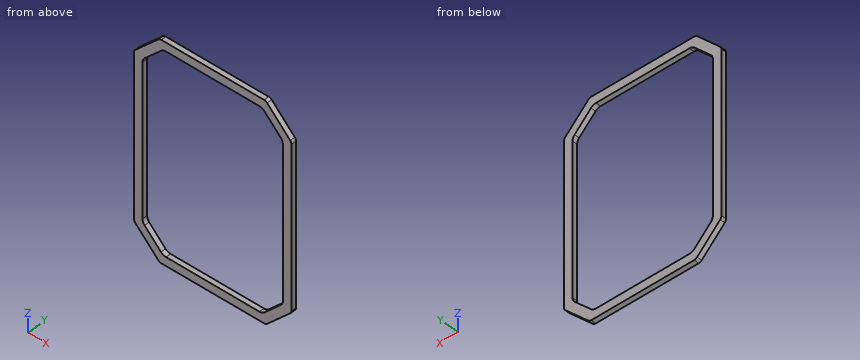
```python
from build123d import *

# Parameters (mm, degrees)
BOSS_EXTRUDE1_DEPTH = 1.75


with BuildPart() as part:
    # Sketch1 → Boss-Extrude1 (new body)
    with BuildSketch(Plane(origin=(-905.783657891, 0, -1752.480725949), x_dir=(1, 0, 0), z_dir=(0, 1, 0))):
        with BuildLine():
            Line((5.86809467, -1.289791394), (-2.192922636, -9.3508087))
            ThreePointArc((-2.192922636, -9.3508087), (-2.518081763, -9.837443723), (-2.632262464, -10.411468871))
            Line((-2.632262464, -10.411468871), (-2.632262464, -66.28943426))
            ThreePointArc((-2.632262464, -66.28943426), (-2.518081763, -66.863459408), (-2.192922636, -67.350094431))
            Line((-2.192922636, -67.350094431), (5.86809467, -75.411111737))
            ThreePointArc((5.86809467, -75.411111737), (6.354729693, -75.736270864), (6.928754842, -75.850451566))
            Line((6.928754842, -75.850451566), (42.80672023, -75.850451566))
            ThreePointArc((42.80672023, -75.850451566), (43.380745379, -75.736270864), (43.867380402, -75.411111737))
            Line((43.867380402, -75.411111737), (51.928397708, -67.350094431))
            ThreePointArc((51.928397708, -67.350094431), (52.253556835, -66.863459408), (52.367737536, -66.28943426))
            Line((52.367737536, -66.28943426), (52.367737536, -10.411468871))
            ThreePointArc((52.367737536, -10.411468871), (52.253556835, -9.837443723), (51.928397708, -9.3508087))
            Line((51.928397708, -9.3508087), (43.867380402, -1.289791394))
            ThreePointArc((43.867380402, -1.289791394), (43.380745379, -0.964632267), (42.80672023, -0.850451566))
            Line((42.80672023, -0.850451566), (6.928754842, -0.850451566))
            ThreePointArc((6.928754842, -0.850451566), (6.354729693, -0.964632267), (5.86809467, -1.289791394))
        make_face()
        with BuildLine():
            Line((6.817842138, -4.582684613), (1.099970583, -10.300556168))
            ThreePointArc((1.099970583, -10.300556168), (0.558038705, -11.11161454), (0.367737536, -12.068323121))
            Line((0.367737536, -12.068323121), (0.367737536, -64.63258001))
            ThreePointArc((0.367737536, -64.63258001), (0.558038705, -65.589288591), (1.099970583, -66.400346963))
            Line((1.099970583, -66.400346963), (6.817842138, -72.118218519))
            ThreePointArc((6.817842138, -72.118218519), (7.62890051, -72.660150397), (8.585609091, -72.850451566))
            Line((8.585609091, -72.850451566), (41.149865981, -72.850451566))
            ThreePointArc((41.149865981, -72.850451566), (42.106574562, -72.660150397), (42.917632934, -72.118218519))
            Line((42.917632934, -72.118218519), (48.635504489, -66.400346963))
            ThreePointArc((48.635504489, -66.400346963), (49.177436367, -65.589288591), (49.367737536, -64.63258001))
            Line((49.367737536, -64.63258001), (49.367737536, -12.068323121))
            ThreePointArc((49.367737536, -12.068323121), (49.177436367, -11.11161454), (48.635504489, -10.300556168))
            Line((48.635504489, -10.300556168), (42.917632934, -4.582684613))
            ThreePointArc((42.917632934, -4.582684613), (42.106574562, -4.040752734), (41.149865981, -3.850451566))
            Line((41.149865981, -3.850451566), (8.585609091, -3.850451566))
            ThreePointArc((8.585609091, -3.850451566), (7.62890051, -4.040752734), (6.817842138, -4.582684613))
        make_face(mode=Mode.SUBTRACT)
    extrude(amount=BOSS_EXTRUDE1_DEPTH)


solid = part.part
```
The model under review builds one solid part; all positions refer to its coordinate system, in mm. Round coordinates to 2 decimals unless told otherwise and drop trailing zeros. Order: outer loops, then holes, each group sorted by start corner. A loop starts at its lowest first (then second) coordinate and runs counter-clockwise, first axis right, second up. Notation, with made-up numbers: M -13,-13.75 L 26,-13.75 A25 ccw 26,10.25 Z; hole C 43,-18 d6. An arc over 180 degrees is marked long. Use a Markdown table: item, result.
1) Consider section B-B (x = -871). Write out the cut boundary in (y, z), then the cut area to 3 significant figures.
Report:
| item | result |
|---|---|
| outline | M 0,-1751.63 L 1.75,-1751.63 L 1.75,-1748.63 L 0,-1748.63 Z; M 0,-1679.63 L 1.75,-1679.63 L 1.75,-1676.63 L 0,-1676.63 Z |
| area | 10.5 mm^2 |
2) Wall thickness on line 1 along Z through (x, y) = (-893, 0.9); line 2 along X through (y, z) = (1.15, -1739); line 3 along Z through (x, y) = (-860, 0.85): over which ranges is each line inside the solid? List them lowest first. Write a range as [from, to].
Report:
| item | result |
|---|---|
| line 1 | [-1751.63, -1748.63], [-1679.63, -1676.63] |
| line 2 | [-908.42, -905.42], [-856.42, -853.42] |
| line 3 | [-1749.27, -1745.03], [-1683.23, -1678.99] |
3) Consider section A-A (z = -1738). Write out the cut boundary in (x, y).
Report:
| item | result |
|---|---|
| outline | M -908.42,0 L -905.42,0 L -905.42,1.75 L -908.42,1.75 Z; M -856.42,0 L -853.42,0 L -853.42,1.75 L -856.42,1.75 Z |
